Here's the drawing with two shaded views (mm, measured from the low corner). I have some questions. A direction names the side the tool comes from. Coordinates: 2 decimals unless noted, no trailing zeros. Order: outer loops, then holes, each group sorted by start corner. A loop starts at its lowest first (then second) coordinate and runs counter-clockwise, first axis right, second up. Notation, with made-up numbers: (48.25, 27) - (62.25, 27) arc R10 cw to (62.25, 38) - close; hole circle Ø5 at (1, 79.5). An arc over 180 degrees is marked (long way). Answer as a JSON object with one key per item and string values. Group by question number.
(1) We'd pull the mould along X, two halves only. Please class the marked faces 1, 2 and 3: pulls with the +X half, pulls with the -X half, needs draft (parallel to the pull), parting line crosses it, or undercut.
(2) Imagine slicing it at C-C, the plane z = 8.25. Write out the boundary of the cut face in (x, y).
(3) Which directions (+Z, -Z, +X, -X, +Y, -Y) give clear straight access to the entire face, cutting with the end or side of a thin tool? Please do the marked faces 4 and 5.
(4) Will these pins go through, and if not, where does the flat tip stop? P1, Ø8, axis at x = 18.5, z = 8.5, coming from the +Y side; P2, Ø6, axis at y = 5, z = 12, coming from the +X side; P3, Ø4, axis at x = 21.5, z = 3.5, coming from the +Y side (1 decimal).
(5) Please list where these lines run through material, in increasing order: probe 1 along X at (y, z) = (12.7, 10.4); probe 2 along Z at (x, y) = (1.5, 13.5).
(6) Imagine slicing it at D-D, the plane z = 3. Write out the boundary of the cut face in (x, y).
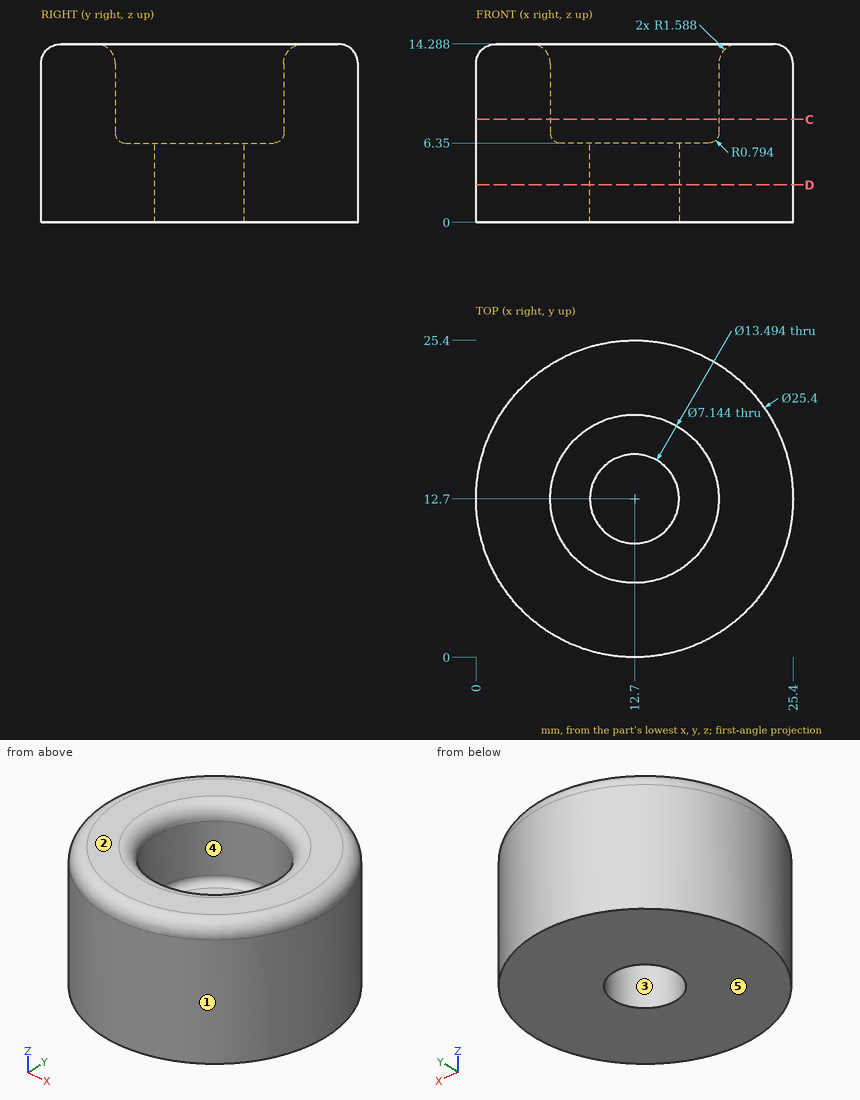
Result set:
{
 "1": {"face 1": "parting line crosses it", "face 2": "needs draft", "face 3": "undercut"},
 "2": {"outline": "circle Ø25.4 at (12.7, 12.7); hole circle Ø13.49 at (12.7, 12.7)"},
 "3": {"face 4": "+Z", "face 5": "-Z, +X, -X, +Y, -Y"},
 "4": {"P1": "stops at y = 25.27", "P2": "stops at x = 24.5", "P3": "stops at y = 23.4"},
 "5": {"probe 1": "x = 0 to 5.95, 19.45 to 25.4", "probe 2": "z = 0 to 14.28"},
 "6": {"outline": "circle Ø25.4 at (12.7, 12.7); hole circle Ø7.14 at (12.7, 12.7)"}
}
